Autodesk Inventor part; units mm, degrees
ref_plane "YZ Plane" through (0, 0, 0) normal (1, 0, 0) x (0, 1, 0)
ref_plane "XZ Plane" through (0, 0, 0) normal (0, 1, 0) x (-1, 0, 0)
ref_plane "XY Plane" through (0, 0, 0) normal (0, 0, 1) x (1, 0, 0)
sketch "Sketch1" plane through (0, 0, 0) normal (0, 1, 0) x (-1, 0, 0)
  line L0 (47.625, 38.1) -> (-47.625, 38.1)
  line L1 (-47.625, 38.1) -> (-47.625, -38.1)
  line L2 (-47.625, -38.1) -> (47.625, -38.1)
  line L3 (47.625, -38.1) -> (47.625, 38.1)
  line L4 (47.625, 38.1) -> (-47.625, -38.1) construction
  line L5 (-47.625, 38.1) -> (47.625, -38.1) construction
  point P0 (0, 0)
  dimension "d0" = 95.25
  dimension "d1" = 76.2
extrude "Extrusion1" add sketch "Sketch1" against normal blind 6.35
sketch "Sketch4" plane through (0, 0, 0) normal (0, 1, 0) x (1, 0, 0)
  line L0 (-47.625, -19.05) -> (-28.575, -19.05)
  line L1 (-28.575, -19.05) -> (-28.575, 19.05)
  line L2 (-28.575, 19.05) -> (-47.625, 19.05)
  line L3 (-47.625, 19.05) -> (-47.625, -19.05)
  line L4 (-47.625, -19.05) -> (-28.575, 19.05) construction
  line L5 (-28.575, -19.05) -> (-47.625, 19.05) construction
  line L6 (-47.625, 38.1) -> (-47.625, -38.1)
  line L7 (-44.45, -15.875) -> (-31.75, -15.875)
  line L8 (-31.75, -15.875) -> (-31.75, 15.875)
  line L9 (-31.75, 15.875) -> (-44.45, 15.875)
  line L10 (-44.45, 15.875) -> (-44.45, -15.875)
  line L11 (-44.45, -15.875) -> (-31.75, 15.875) construction
  line L12 (-31.75, -15.875) -> (-44.45, 15.875) construction
  point P0 (0, 0)
  point P1 (-38.1, 0)
  dimension "d8" = 0
  dimension "d9" = 38.1
  dimension "d10" = 19.05
  dimension "d11" = 3.175
  dimension "d12" = 3.175
extrude "Extrusion2" add sketch "Sketch4" along normal blind 153.924
sketch "Sketch5" plane through (-47.625, -6.35, -38.1) normal (-1, 0, 0) x (0, 0, 1)
  circle A0 centre (38.1, 84.074) radius 4.7625
  line L0 (19.05, 160.274) -> (57.15, 160.274)
  point P0 (38.1, 6.35)
  dimension "d15" = 9.525
  dimension "d16" = 76.2
extrude "Extrusion3" cut sketch "Sketch5" against normal through all
equation "\"d0\" = baseWidth"
equation "\"d1\" = baseLength"
equation "\"d2\" = baseThickness"
equation "\"d9\" = postLength"
equation "\"d10\" = postWidth"
equation "\"d11\" = postWallThickness"
equation "\"d12\" = postWallThickness"
equation "\"d13\" = postHeight"
equation "\"d15\" = postAxelDiam"
equation "\"d16\" = heightFromTopToAxelCenter"
equation "\"d17\" = postHeight"
equation "\"baseWidth\" = 95.25"
equation "\"baseLength\" = 76.2"
equation "\"baseThickness\" = 6.35"
equation "\"postWidth\" = 19.05"
equation "\"postLength\" = 38.1"
equation "\"postWallThickness\" = 3.175"
equation "\"postHeight\" = 153.924"
equation "\"postAxelDiam\" = 9.525"
equation "\"heightFromTopToAxelCenter\" = 76.2"
properties part number "BasePostForSideOfRobot"
Work out the finished part from the listing and answer in its coordinate system (mm). A direction names the side the tool comes from. Round coordinates to 2 decimals unless told otherwise and drop trailing zeros. Write each loop counter-clockwise with the first axis right and the second up, starting at its lowest first coordinate (ties: lowest second). Pieces come first, ordered by that corner, then holes.
1) A cutting plane is placed at C-C on z = -9. Determine the outline of the cut face in (x, y) (3 decimals), and give its area (3 significant figures).
2) Flat-ended cylindrical pins translate along their axes: P1, Ø6, axis at y = 131.5, z = 0.5, coming from the +X side (3 decimals); P2, Ø4, axis at x = -41, y = 77.5, coming from the +Z side; P3, Ø15, axis at x = -34, y = 69.5, coming from the -Z side. Find the tip coordinate at first contact, or state that the pin passes through.
3) Determine the mould class of faces 1 (the face through (-45, 153.924, 0)), 2 (the face through (-44.45, 76, 7)), 3 (the face through (-30.185, 73.075, -1.032)) for opening direction Y: pulls with the +Y half, pulls with the -Y half, needs draft (parallel to the pull), parting line crosses it, or undercut.
4) Which of the six approach directions +Z, -Z, +X, -X, +Y, -Y give full straight-line access (tool end or side, diameter ignored) to faces 4 (the face through (-38, 76, -19.05)), 5 (the face through (-38, 76, -15.875)), 6 (the face through (-38, 76, 19.05))?
5) A cutting plane is placed at D-D on x = 22. Determine the outline of the cut face in (y, z).
6) A cutting plane is placed at A-A on z = 0. Give the number of separate pieces and of enclosed holes in the cut face, and give its area (3 significant figures).
7) A cutting plane is placed at B-B on y = 119. Determine the outline of the cut face in (x, z) (3 decimals).
8) Consider probe 1 along Y at (x, z) = (-46, 0); probe 2 along X at (y, z) = (17, 13.5) (3 decimals); probe 3 along Y at (x, z) = (-9, -18). Determine where each line is inside the solid, lowest interval first.
Entries:
1. outline: (-47.625, -6.35) - (47.625, -6.35) - (47.625, 0) - (-28.575, 0) - (-28.575, 153.924) - (-31.75, 153.924) - (-31.75, 0) - (-44.45, 0) - (-44.45, 153.924) - (-47.625, 153.924) - close
1. area: 1,580 mm2
2. P1: stops at x = -28.575
2. P2: stops at z = 19.05
2. P3: stops at z = -19.05
3. face 1: pulls with the +Y half
3. face 2: needs draft
3. face 3: undercut
4. face 4: -Z, +X, -X, +Y
4. face 5: +Y
4. face 6: +Z, +X, -X, +Y
5. outline: (-6.35, -38.1) - (0, -38.1) - (0, 38.1) - (-6.35, 38.1) - close
6. separate pieces: 3
6. enclosed holes: 0
6. area: 1,520 mm2
7. outline: (-47.625, -19.05) - (-28.575, -19.05) - (-28.575, 19.05) - (-47.625, 19.05) - close; hole (-44.45, -15.875) - (-31.75, -15.875) - (-31.75, 15.875) - (-44.45, 15.875) - close
8. probe 1: y = -6.35 to 72.96, 82.49 to 153.92
8. probe 2: x = -47.625 to -44.45, -31.75 to -28.575
8. probe 3: y = -6.35 to 0
